from build123d import *

# Parameters (mm, degrees)
SKIZZE1_W                       = 275
SKIZZE1_H                       = 150
SKIZZE1_R                       = 1.65
SKIZZE1_R_2                     = 17.75
SKIZZE1_W_2                     = 179.5
SKIZZE1_H_2                     = 59
SKIZZE1_W_3                     = 47
SKIZZE1_H_3                     = 38
AUFSATZ_LINEAR_AUSTRAGEN1_DEPTH = 3


with BuildPart() as part:
    # Skizze1 → Aufsatz-Linear austragen1 (new body)
    with BuildSketch(Plane(origin=(0, 0, 0), x_dir=(1, 0, 0), z_dir=(0, 1, 0))):
        Rectangle(SKIZZE1_W, SKIZZE1_H)
        with Locations(Location((-129.5, -67, 0), (0, 0, 270))):
            Circle(SKIZZE1_R, mode=Mode.SUBTRACT)
        with Locations(Location((129.5, -67, 0), (0, 0, 270))):
            Circle(SKIZZE1_R, mode=Mode.SUBTRACT)
        with Locations(Location((-129.5, 67, 0), (0, 0, 270))):
            Circle(SKIZZE1_R, mode=Mode.SUBTRACT)
        with Locations(Location((129.5, 67, 0), (0, 0, 270))):
            Circle(SKIZZE1_R, mode=Mode.SUBTRACT)
        with Locations(Location((25.525, -26.5, 0), (0, 0, 270))):
            Circle(SKIZZE1_R_2, mode=Mode.SUBTRACT)
        with Locations((-0.375, 29)):
            Rectangle(SKIZZE1_W_2, SKIZZE1_H_2, mode=Mode.SUBTRACT)
        with Locations((-27.875, -26.15)):
            Rectangle(SKIZZE1_W_3, SKIZZE1_H_3, mode=Mode.SUBTRACT)
    extrude(amount=AUFSATZ_LINEAR_AUSTRAGEN1_DEPTH)


solid = part.part
Could you check a few things on this model? Use its own coordinates, in mm. Round coordinates to 2 decimals unless told otherwise and drop trailing zeros. Order: outer loops, then holes, each group sorted by start corner. A loop starts at its lowest first (then second) coordinate and runs counter-clockwise, first axis right, second up.
(1) Imagine slicing it at A-A (x = 74). Write out the boundary of the cut face in (y, z).
Response values:
outline: (0, -75) - (3, -75) - (3, -58.5) - (0, -58.5) - close; (0, 0.5) - (3, 0.5) - (3, 75) - (0, 75) - close
(2) I'm going to push a flat-ended pin straight in: pin 1 (4 mm diameter, centred on x = -129.5, z = -67, fed in from +Y). Where does the tip first touch, or does it pass through?
Response values:
pin 1: stops at y = 3
(3) Imagine slicing it at D-D (z = 26.5). Write out the boundary of the cut face in (x, y) (3 decimals), plus the area to 4 significant figures.
Response values:
outline: (-137.5, 0) - (-51.375, 0) - (-51.375, 3) - (-137.5, 3) - close; (-4.375, 0) - (7.775, 0) - (7.775, 3) - (-4.375, 3) - close; (43.275, 0) - (137.5, 0) - (137.5, 3) - (43.275, 3) - close
area: 577.5 mm2
(4) Please list where these lines run through material, in increasing order: line 1 along Z through (x, y) = (129.5, 1.25); line 2 along X through (y, z) = (1.85, 26.5) (3 decimals); line 3 along Z through (x, y) = (-15, 1.8).
Response values:
line 1: z = -75 to -68.65, -65.35 to 65.35, 68.65 to 75
line 2: x = -137.5 to -51.375, -4.375 to 7.775, 43.275 to 137.5
line 3: z = -75 to -58.5, 0.5 to 7.15, 45.15 to 75
(5) If we mould it in two halves opening along Z, with no side actions, what happens to faces 1 (the flat face through (-2, 0, 16)), 2 (the cylindrical face through (30.86, 1.48, 43.43))? For each: released by +Z, released by -Z, zero draft, split by the parting line, or undercut.
Response values:
face 1: zero draft
face 2: undercut
(6) Imagine slicing it at C-C (x = -48.5). Write out the boundary of the cut face in (y, z).
Response values:
outline: (0, -75) - (3, -75) - (3, -58.5) - (0, -58.5) - close; (0, 0.5) - (3, 0.5) - (3, 7.15) - (0, 7.15) - close; (0, 45.15) - (3, 45.15) - (3, 75) - (0, 75) - close
(7) Imagine slicing it at B-B (z = -22.5). Write out the boundary of the cut face in (x, y) (3 decimals).
Response values:
outline: (-137.5, 0) - (-90.125, 0) - (-90.125, 3) - (-137.5, 3) - close; (89.375, 0) - (137.5, 0) - (137.5, 3) - (89.375, 3) - close
